CAD build for the part. Positions are in the model's coordinates, mm. A direction names the side the tool comes from. Give positions to 0.01 mm unless a question says otherwise; leave off trailing zeros. Order: outer loops, then holes, each group sorted by start corner. A loop starts at its lowest first (then second) coordinate and runs counter-clockwise, first axis right, second up.
Item 1: Wall check: L1, parallel to X at y = 8, z = 0; L2, parallel to X at y = 11.25, z = 5.5; L3, parallel to X at y = 1.5, z = -1. Give the ranges that are in metal, low to high.
Item 2: Flat gauge pins, fed straight in: P1, Ø23, axis at x = 25, z = 0, coming from the +Y side; P2, Ø10, axis at x = 31.5, y = 4.5, coming from the -Z side; P3, Ø2, axis at x = 22.5, y = 8, coming from the -Z side; P4, Ø5, axis at x = 27, y = 13.5, coming from the +Z side. Where does each tip first touch, or does it go through?
Item 3: Band-saw the part on C-C on x = 25. Give the cut face in (y, z), plus the area to 3 significant figures.
Item 4: Band-saw the part on B-B on y = 12.5. Give the cut face in (x, z).
Item 5: Which spindle directions (+Z, -Z, +X, -X, +Y, -Y) get a long thin tool onto all of the face, cutting with end or side? Do faces 1 (the flat face through (-1, 20, 11)), 2 (the flat face through (0, 10, 2)). Say none if no direction does.
Item 6: Band-saw the part on D-D on z = 20.5. Give the cut face in (x, y), plus the area to 3 significant figures.
Item 7: Two-plate mould, pull along X, no slides. Class faces 3 (the cylindrical face through (50.334, 9.86, -15.851)), 4 (the flat face through (-1, 0, 11)), 5 (the cylindrical face through (-15.46, 10.14, -3)): released by +X, released by -X, zero draft, split by the parting line, or undercut.
Item 8: Band-saw the part on A-A on z = 0. Give the cut face in (x, y).
```python
from build123d import *

# Parameters (mm, degrees)
SKETCH1_R           = 52.771281292
BOSS_EXTRUDE1_DEPTH = 20
SKETCH3_R           = 10
CUT_EXTRUDE1_DEPTH  = 20


with BuildPart() as part:
    # Sketch1 → Boss-Extrude1 (new body)
    with BuildSketch(Plane(origin=(0, 0, 0), x_dir=(1, 0, 0), z_dir=(0, 1, 0))):
        Circle(SKETCH1_R)
        with BuildLine():
            Line((-1.918332609, -2), (1.918332609, -2))
            ThreePointArc((1.918332609, -2), (0, 2.771281292), (-1.918332609, -2))
        make_face(mode=Mode.SUBTRACT)
    extrude(amount=BOSS_EXTRUDE1_DEPTH)

    # Sketch3 → Cut-Extrude1 (cut)
    with BuildSketch(Plane(origin=(0, 20, 0), x_dir=(1, 0, 0), z_dir=(0, 1, 0))):
        with Locations((-25, 0)):
            Circle(SKETCH3_R)
        with Locations((0, 25)):
            Circle(SKETCH3_R)
        with Locations((25, 0)):
            Circle(SKETCH3_R)
        with Locations((0, -25)):
            Circle(SKETCH3_R)
    extrude(amount=-CUT_EXTRUDE1_DEPTH, mode=Mode.SUBTRACT)


solid = part.part
```
The answers:
1. L1: x = -52.77 to -35, -15 to -2.77, 2.77 to 15, 35 to 52.77
1. L2: x = -52.48 to -33.35, -16.65 to 16.65, 33.35 to 52.48
1. L3: x = -52.76 to -34.95, -15.05 to -2.58, 2.58 to 15.05, 34.95 to 52.76
2. P1: stops at y = 20
2. P2: stops at z = -45.64
2. P3: stops at z = -48.19
2. P4: stops at z = 46.74
3. outline: (0, -46.47) - (20, -46.47) - (20, -10) - (0, -10) - close; (0, 10) - (20, 10) - (20, 46.47) - (0, 46.47) - close
3. area: 1,460 mm2
4. outline: circle Ø105.54 at (0, 0); hole circle Ø20 at (-25, 0); hole circle Ø20 at (0, -25); hole circle Ø20 at (0, 25); hole (-1.92, 2) arc R2.77 ccw (long way) to (1.92, 2) - close; hole circle Ø20 at (25, 0)
5. face 1: +Z, -Z, +X, -X, +Y
5. face 2: +Y, -Y
6. outline: (-48.63, 0) - (-8.93, 0) - (-8.93, 20) - (-48.63, 20) - close; (8.93, 0) - (48.63, 0) - (48.63, 20) - (8.93, 20) - close
6. area: 1,590 mm2
7. face 3: split by the parting line
7. face 4: zero draft
7. face 5: undercut
8. outline: (-52.77, 0) - (-35, 0) - (-35, 20) - (-52.77, 20) - close; (-15, 0) - (-2.77, 0) - (-2.77, 20) - (-15, 20) - close; (2.77, 0) - (15, 0) - (15, 20) - (2.77, 20) - close; (35, 0) - (52.77, 0) - (52.77, 20) - (35, 20) - close
